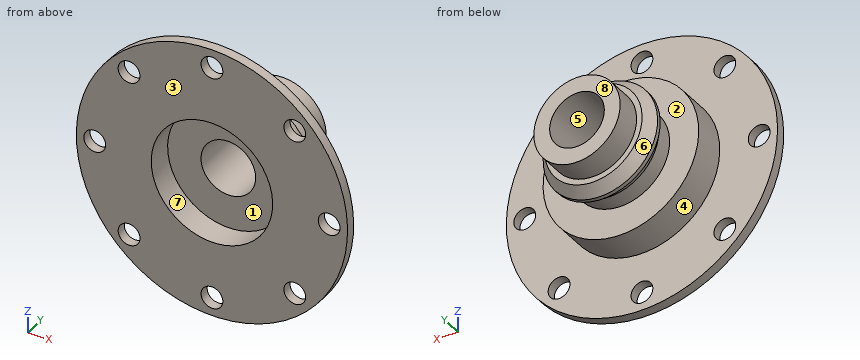
```python
from build123d import *

# Parameters (mm, degrees)
F2_R     = 4
F3_DEPTH = 254


with BuildPart() as f1:
    # F0 (on Right) → F1 (revolve)
    with BuildSketch(Plane.YZ):
        Polygon((0, 49.75), (0, 22.275), (9.5, 22.275), (9.5, 10.0325), (41.2, 10.0325), (41.2, 15.85), (31.7, 15.85), (31.7, 17.875), (27.65, 21), (26.15, 21), (22.1, 17.875), (15.75, 17.875), (15.75, 28.55), (3.55, 28.55), (3.55, 49.75), align=None)
    revolve(axis=Axis((0, 2500.943971, 0), (0, 1, 0)))

    # F2 (on face) → F3 (cut, symmetric)
    with BuildSketch(Plane(origin=(0, 3.55, 0), x_dir=(-1, 0, 0), z_dir=(0, 1, 0))):
        with Locations((0, 43)):
            Circle(F2_R)
        with Locations((-30.405592, 30.405592)):
            Circle(F2_R)
        with Locations((43, 0)):
            Circle(F2_R)
        with Locations((30.405592, 30.405592)):
            Circle(F2_R)
        with Locations((-30.405592, -30.405592)):
            Circle(F2_R)
        with Locations((-43, 0)):
            Circle(F2_R)
        with Locations((0, -43)):
            Circle(F2_R)
        with Locations((30.405592, -30.405592)):
            Circle(F2_R)
    extrude(amount=F3_DEPTH, both=True, mode=Mode.SUBTRACT)


solid = f1.part
```
For this review, take the finished solid that the model builds, in its own axes (mm). Face numbers are marked on the shaded views. A direction names the side the tool comes from. Round coordinates to 2 decimals unless told otherwise and drop trailing zeros. Order: outer loops, then holes, each group sorted by start corner. A loop starts at its lowest first (then second) coordinate and runs counter-clockwise, first axis right, second up.
Q1. Wall thickness on line 1 (X direction, y = 3.5, z = -31.5); line 2 (X direction, y = 4, z = 0) (3 decimals); line 3 (X direction, y = 27, z = 0): over which ranges is each line inside the solid? List them lowest first.
Findings below:
line 1: x = -38.51 to -34.25, -26.56 to 26.56, 34.25 to 38.51
line 2: x = -28.55 to -22.275, 22.275 to 28.55
line 3: x = -21 to -10.03, 10.03 to 21
Q2. Machinability: for the marked faces 1, 2, 3 and 4, which of the approach directions +Z, -Z, +X, -X, +Y, -Y give a long, thin tool a straight path to every point of the face, cutting with its end or side? Answer none if there is none.
Findings below:
face 1: -Y
face 2: none
face 3: +Z, -Z, +X, -X, -Y
face 4: +Y
Q3. We need section D-D, the plane x = -43. Give the boundary of the cut face in (y, z).
Findings below:
outline: (0, -25.02) - (3.55, -25.02) - (3.55, -4) - (0, -4) - close; (0, 4) - (3.55, 4) - (3.55, 25.02) - (0, 25.02) - close
Q4. We need section B-B, the plane x = -33. Give the boundary of the cut face in (y, z), plus the area to 3 significant figures.
Findings below:
outline: (0, -37.23) - (3.55, -37.23) - (3.55, -33.45) - (0, -33.45) - close; (0, -27.36) - (3.55, -27.36) - (3.55, 27.36) - (0, 27.36) - close; (0, 33.45) - (3.55, 33.45) - (3.55, 37.23) - (0, 37.23) - close
area: 221 mm2
Q5. Insertion check: P1, Ø6.5, axis at x = 0, z = -43, coming from the -Y side; P2, Ø9, axis at x = 30.41, z = 30.41, coming from the +Y side; P3, Ø2, axis at x = -10, z = -18.5, coming from the +Y side; P4, Ø6, axis at y = 6, z = 4.5, coming from the +X side. Each pin has a flat end and moves straight along its axis. Give the tip position at first contact, or say it passes through.
Findings below:
P1: passes through
P2: stops at y = 3.55
P3: stops at y = 28.91
P4: stops at x = 49.67
Q6. Mouldability with a two-part tool opening along X and no side actions: class the marked faces 5, 6, 7 and 8 as pulls with the +X half, pulls with the -X half, needs draft (parallel to the pull), parting line crosses it, or undercut.
Findings below:
face 5: undercut
face 6: parting line crosses it
face 7: undercut
face 8: needs draft
Q7. We need section C-C, the plane z = 43. Give the boundary of the cut face in (x, y).
Findings below:
outline: (-25.02, 0) - (-4, 0) - (-4, 3.55) - (-25.02, 3.55) - close; (4, 0) - (25.02, 0) - (25.02, 3.55) - (4, 3.55) - close
